Geometry: final body of the model. Coordinates: model frame, mm. Face numbers are marked on the shaded views. A direction names the side the tool comes from. Give positions to 0.01 mm unless a question says otherwise; leave off trailing zeros. Write each loop counter-clockwise with the first axis right and the second up, starting at its lowest first coordinate (ties: lowest second). Pieces come first, ordered by that corner, then holes. Notation, with made-up numbers: M -33,-14 L -24,-14 A17 cw -24,-6 Z; hole C 26.25,53.25 d9. An arc over 180 degrees is marked long. Use one line per item in the form item = value. Start each with the question number.
Item 1: Pull-direction query (Y, two-part tool) for the marked faces 1, 2 and 3; classes: released by +Y, released by -Y, zero draft, split by the parting line, or undercut.
Item 2: Section query A-A on y = -19.05. Return loops of the section in (x, z), then the cut area to 3 significant figures.
Item 3: Material intervals for line 1 along X through (y, z) = (-19, -10); line 2 along Z through (x, y) = (18, -21); line 3 along Z through (x, y) = (52.5, -3.5), sorted ascending. Write a range as from..to.
Item 4: Access query for the marked faces 4, 5, 6, 7 and 8. Directions: +Z, -Z, +X, -X, +Y, -Y. A direction counts if a zero-diameter tool reaches every point of the face in a straight line with its end or side. Return the directions, or none.
Item 5: Section query B-B on x = 21.5. Return loops of the section in (y, z), then the cut area to 3 significant figures.
Item 6: Contact query for flat-ended pins moving along their axis: P1, Ø8, axis at x = -21.5, y = -62.5, coming from the +Z side; P2, Ø10.5, axis at y = -19, z = -1.5, coming from the +X side; P3, Ø8, axis at y = -16.5, z = 10, coming from the +X side; P4, Ø2, axis at y = -42.5, z = 19.5, coming from the -X side. Output: stop coordinate, or through.
Item 7: Section query C-C on y = -46. Return loops of the section in (x, z).
Item 8: Section query D-D on z = 31. Return loops of the section in (x, y), then the cut area to 3 significant figures.
from build123d import *

# Parameters (mm, degrees)
F0_W      = 120.65
F0_H      = 12.7
F1_DEPTH  = 69.85
F2_R      = 7.874
F3_DEPTH  = 15.748
F5_DEPTH  = 12.7
F4_W      = 44.45
F4_H      = 47.498
F6_DEPTH  = 40.894
F7_W      = 47.498
F7_H      = 22.098
F8_DEPTH  = 25.4
F9_W      = 15.748
F9_H      = 19.05
F10_DEPTH = 44.45


with BuildPart() as f1:
    # F0 (on Front) → F1 (new body)
    with BuildSketch(Plane.XZ):
        with Locations((0.915147, -11.16853)):
            Rectangle(F0_W, F0_H)
    extrude(amount=F1_DEPTH)

    # F2 (on face) → F3 (cut)
    with BuildSketch(Plane.XY.offset(-4.81853)):
        with Locations((42.190147, -19.05)):
            Circle(F2_R)
        with Locations((-40.359853, -19.05)):
            Circle(F2_R)
    extrude(amount=-F3_DEPTH, mode=Mode.SUBTRACT)

    # F2 (on face) → F5 (cut)
    with BuildSketch(Plane.XY.offset(-4.81853)):
        Polygon((-59.409853, -69.85), (-21.309853, -69.85), (-59.409853, -31.75), align=None)
        Polygon((61.240147, -69.85), (61.240147, -31.75), (23.140147, -69.85), align=None)
    extrude(amount=-F5_DEPTH, mode=Mode.SUBTRACT)

    # F4 (on face) → F6 (join)
    with BuildSketch(Plane.XY.offset(-4.81853)):
        with Locations((0.915147, -23.749)):
            Rectangle(F4_W, F4_H)
    extrude(amount=F6_DEPTH)

    # F7 (on face) → F8 (cut)
    with BuildSketch(Plane.YZ.offset(23.140147)):
        with Locations((-23.749, 15.62847)):
            Rectangle(F7_W, F7_H)
    extrude(amount=-F8_DEPTH, mode=Mode.SUBTRACT)

    # F9 (on face) → F10 (cut)
    with BuildSketch(Plane(origin=(-21.309853, 0, 0), x_dir=(0, -1, 0), z_dir=(-1, 0, 0))):
        with Locations((39.624, 26.55047)):
            Rectangle(F9_W, F9_H)
    extrude(amount=-F10_DEPTH, mode=Mode.SUBTRACT)


solid = f1.part
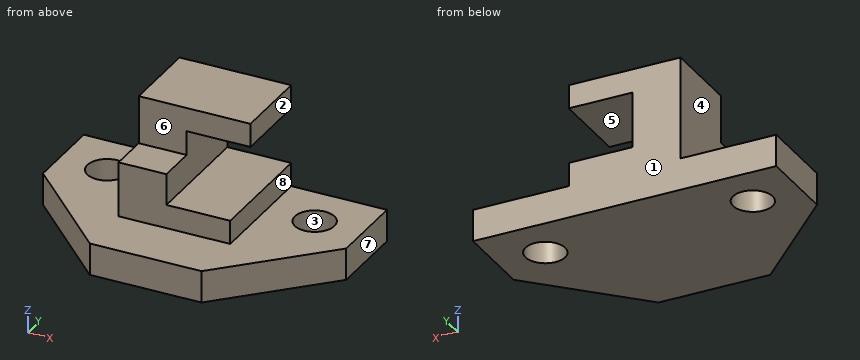
Answer sheet:
q1.face_1 = released by +Y
q1.face_2 = zero draft
q1.face_3 = undercut
q2.outline = M -59.41,-17.52 L -48.23,-17.52 L -48.23,-4.82 L -59.41,-4.82 Z; M -32.49,-17.52 L 34.32,-17.52 L 34.32,-4.82 L 23.14,-4.82 L 23.14,4.58 L -2.26,4.58 L -2.26,26.68 L 23.14,26.68 L 23.14,36.08 L -21.31,36.08 L -21.31,-4.82 L -32.49,-4.82 Z; M 50.06,-17.52 L 61.24,-17.52 L 61.24,-4.82 L 50.06,-4.82 Z
q2.area = 2,390 mm2
q3.line_1 = -59.41..-48.23, -32.49..34.32, 50.06..61.24
q3.line_2 = -17.52..4.58, 26.68..36.08
q3.line_3 = -17.52..-4.82
q4.face_4 = +Z, -X, +Y, -Y
q4.face_5 = +X, +Y, -Y
q4.face_6 = +Z, +X, -X, -Y
q4.face_7 = +Z, -Z, +X, +Y, -Y
q4.face_8 = +Z, +X, +Y, -Y
q5.outline = M -69.85,-17.52 L 0,-17.52 L 0,4.58 L -47.5,4.58 L -47.5,-4.82 L -69.85,-4.82 Z; M -31.75,26.68 L 0,26.68 L 0,36.08 L -31.75,36.08 Z
q5.area = 1,630 mm2
q6.P1 = -4.82
q6.P2 = 61.24
q6.P3 = -2.26
q6.P4 = through
q7.outline = M -45.16,-17.52 L 46.99,-17.52 L 46.99,-4.82 L 23.14,-4.82 L 23.14,4.58 L -2.26,4.58 L -2.26,17.03 L -21.31,17.03 L -21.31,-4.82 L -45.16,-4.82 Z
q8.outline = M -21.31,-31.75 L 23.14,-31.75 L 23.14,0 L -21.31,0 Z
q8.area = 1,410 mm2
